Input: dimensioned drawing with shaded views. Units: mm. Origin: part minimum x, y, z. A direction names the side the tool comes from. Round coordinates to 2 decimals unless told otherwise and drop trailing zeros. Write each loop counter-clockwise with the first axis right and the second up, starting at its lowest first coordinate (ties: lowest second). Pieces come first, ordered by that corner, then holes. Notation, with made-up numbers: M 47,74.5 L 98,74.5 A16 cw 98,87.5 Z; hole C 81,23 d6. An arc over 180 degrees is marked long. Answer in a Markdown table with one row per item. Add a question column.
Item 1: Set-up query: the marked faces 1 and 2. Return all of +Z, -Z, +X, -X, +Y, -Y with unobstructed straight access to the full face (end or side cutting, diameter ignored); none if empty.
Item 2: Material intervals for probe 1 along Z at (x, y) = (5.85, 5.5) (1 decimal); probe 2 along X at (y, z) = (4, 7.5) (1 decimal); probe 3 along Z at (x, y) = (6.5, 11.5) (1 decimal), sorted ascending.
Item 3: Contact query for flat-ended pins moving along their axis: pin 1 (1.5 mm diameter, centred on x = 1.5, y = 4, fed in from -Z); pin 2 (8 mm diameter, centred on y = 5, z = 10, fed in from +X); pin 3 (1 mm diameter, centred on x = 6.5, y = 4.5, fed in from -Z). Output: stop coordinate, or through.
Item 4: Cut plane C-C on z = 6. Return loops of the section in (x, y).
Item 5: Cut plane A-A on x = 4.5. Return loops of the section in (y, z).
Item 6: Cut plane D-D on x = 1.25. Return loops of the section in (y, z) (1 decimal).
Item 7: Mould query, pull axis X, two halves, no side actions, for the marked faces 3, 4, 5 and 6. Classes: released by +X, released by -X, zero draft, split by the parting line, or undercut.
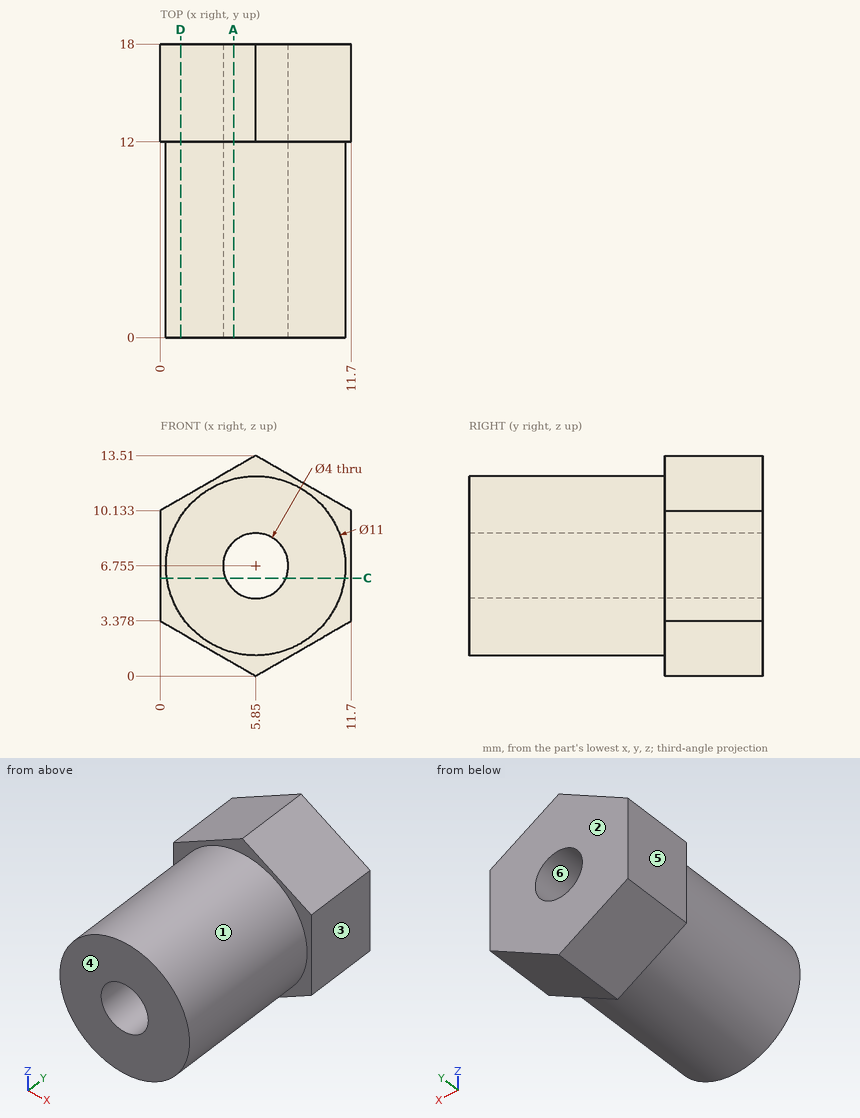
Results below:
| question | item | result |
|---|---|---|
| 1 | face 1 | -Y |
| 1 | face 2 | +Z, -Z, +X, -X, +Y |
| 2 | probe 1 | 1.3 to 4.8, 8.8 to 12.3 |
| 2 | probe 2 | 0.4 to 4, 7.7 to 11.3 |
| 2 | probe 3 | 1.3 to 4.9, 8.6 to 12.2 |
| 3 | pin 1 | z = 2.6 |
| 3 | pin 2 | x = 11.35 |
| 3 | pin 3 | z = 1.26 |
| 4 | outline | M 0,12 L 0.4,12 L 0.4,0 L 4,0 L 4,18 L 0,18 Z; M 7.7,0 L 11.3,0 L 11.3,12 L 11.7,12 L 11.7,18 L 7.7,18 Z |
| 5 | outline | M 0,1.42 L 12,1.42 L 12,0.78 L 18,0.78 L 18,5.28 L 0,5.28 Z; M 0,8.23 L 18,8.23 L 18,12.73 L 12,12.73 L 12,12.09 L 0,12.09 Z |
| 6 | outline | M 0,3.7 L 12,3.7 L 12,2.7 L 18,2.7 L 18,10.9 L 12,10.9 L 12,9.8 L 0,9.8 Z |
| 7 | face 3 | released by +X |
| 7 | face 4 | zero draft |
| 7 | face 5 | released by -X |
| 7 | face 6 | undercut |
